Check sheet for the drawn part. Datum: minimum x, y, z corner. Units: mm. A direction names the side the tool comes from. Give positions to 0.01 mm unless a question says otherwise; leave off trailing zeros. Loops run counter-clockwise (first coordinate to the right, second up) from the corner with the lowest first, then second, coordinate; pieces in that order, holes last.
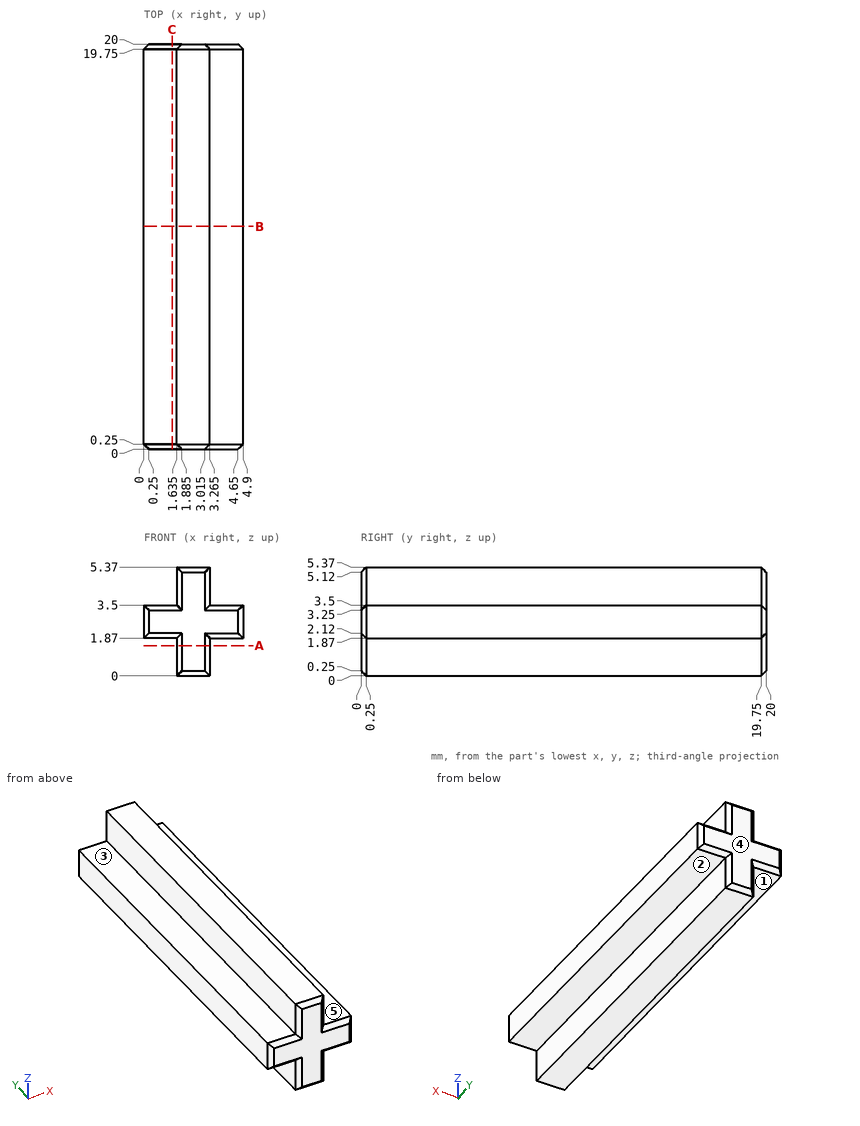
1) Sectioned sample at C-C on x = 1.4. Enter the section's corners in (y, z).
2) Sectioned sample at B-B on y = 11. Enter the section's corners in (x, z) (3 decimals).
3) Scan lines: line 1 along X through (y, z) = (4.75, 1.15) (3 decimals); line 2 along Z through (x, y) = (3.3, 17.5); line 3 along Y through (x, z) = (3.55, 3.4). Record each from-to range of solid material in increasing order.
4) Tool access check on the marked faces 1, 2, 3, 4 and 5. Record the directions out of +Z, -Z, +X, -X, +Y, -Y that give a thin tool (end or side, any length) a straight path to the whole face; none if there is none.
5) Depth check by flat-ended pin: P1, Ø1.3, axis at x = 4, y = 7.5, coming from the +Z side; P2, Ø0.9, axis at y = 14.5, z = 4, coming from the +X side (3 decimals); P3, Ø1.5, axis at y = 9, z = 4.5, coming from the -X side (3 decimals). Enter the tip coordinate at first touch or a pass-through.
6) Sectioned sample at A-A on z = 1.5. Enter the section's corners in (x, y) (3 decimals), plus the area to 3 significant figures.
Determined:
1. outline: (0, 2.12) - (0.25, 1.87) - (19.75, 1.87) - (20, 2.12) - (20, 3.25) - (19.75, 3.5) - (0.25, 3.5) - (0, 3.25) - close
2. outline: (0, 1.87) - (1.635, 1.87) - (1.635, 0) - (3.265, 0) - (3.265, 1.87) - (4.9, 1.87) - (4.9, 3.5) - (3.265, 3.5) - (3.265, 5.37) - (1.635, 5.37) - (1.635, 3.5) - (0, 3.5) - close
3. line 1: x = 1.635 to 3.265
3. line 2: z = 1.87 to 3.5
3. line 3: y = 0.15 to 19.85
4. face 1: -Z, -X, +Y, -Y
4. face 2: -Z, +X, +Y, -Y
4. face 3: +Z, -X, +Y, -Y
4. face 4: +Z, -Z, +X, -X, +Y
4. face 5: +Z, +X, +Y, -Y
5. P1: stops at z = 3.5
5. P2: stops at x = 3.265
5. P3: stops at x = 1.635
6. outline: (1.635, 0.25) - (1.885, 0) - (3.015, 0) - (3.265, 0.25) - (3.265, 19.75) - (3.015, 20) - (1.885, 20) - (1.635, 19.75) - close
6. area: 32.5 mm2
